Autodesk Inventor part; units mm, degrees
ref_plane "YZ Plane" through (0, 0, 0) normal (1, 0, 0) x (0, 1, 0)
ref_plane "XZ Plane" through (0, 0, 0) normal (0, 1, 0) x (-1, 0, 0)
ref_plane "XY Plane" through (0, 0, 0) normal (0, 0, 1) x (1, 0, 0)
sketch "Sketch1" plane through (0, 0, 0) normal (0, 1, 0) x (-1, 0, 0)
  line L0 (0, 0) -> (52.3748, 0) construction
  arc A0 (52.2043, -29.1712) -> (0.1705, -29.1712) centre (26.1874, -26.1874) ccw construction
  line L1 (0, 0) -> (-6.35, 0) construction
  line L2 (52.3748, 0) -> (58.7248, 0) construction
  line L3 (0, 0) -> (0, -26.1874) construction
  line L4 (52.3748, 0) -> (52.3748, -26.1874) construction
  line L5 (-3.175, 0) -> (0.1705, -29.1712)
  line L6 (55.5498, 0) -> (52.2043, -29.1712)
  arc A1 (0.1705, -29.1712) -> (52.2043, -29.1712) centre (26.1874, -26.1874) ccw
  line L7 (-0.0207, 3.5368) -> (52.3955, 3.5368)
  arc A2 (-0.0207, 3.5368) -> (-3.175, 0) centre (-0.0207, 0.3618) ccw
  arc A3 (55.5498, 0) -> (52.3955, 3.5368) centre (52.3955, 0.3618) ccw
  arc A4 (56.8115, -0.1447) -> (52.3955, 4.8068) centre (52.3955, 0.3618) ccw
  line L8 (52.3955, 4.8068) -> (-0.0207, 4.8068)
  arc A5 (-0.0207, 4.8068) -> (-4.4367, -0.1447) centre (-0.0207, 0.3618) ccw
  line L9 (-4.4367, -0.1447) -> (-1.0912, -29.3159)
  arc A6 (-1.0912, -29.3159) -> (53.466, -29.3159) centre (26.1874, -26.1874) ccw
  line L10 (56.8115, -0.1447) -> (53.466, -29.3159)
  dimension "d0" = 52.3748
  dimension "d1" = 52.3748
  dimension "d2" = 6.35
  dimension "d3" = 6.35
  dimension "d4" = 3.175
  dimension "d5" = 1.27
  dimension "d6" = 1.27
  dimension "d7" = 1.27
  dimension "d8" = 1.27
extrude "Extrusion1" add sketch "Sketch1" along normal blind 5.08
properties part number "Clippard Zip Tie 2" material "ABS Plastic"
Model file for the job. Use its own axes, mm. A direction names the side the tool comes from. Round coordinates to 2 decimals unless told otherwise and drop trailing zeros. Loops run counter-clockwise (first coordinate to the right, second up) from the corner with the lowest first, then second, coordinate; pieces in that order, holes last.
1. Band-saw the part on C-C, the plane z = -3.5. List the corners of the cut face in (x, y).
Check values:
outline: (-56.43, 0) - (-55.15, 0) - (-55.15, 5.08) - (-56.43, 5.08) - close; (2.77, 0) - (4.05, 0) - (4.05, 5.08) - (2.77, 5.08) - close
2. Wall check: probe 1 along X at (y, z) = (2.25, -38.5); probe 2 along X at (y, z) = (3.9, -13); probe 3 along Z at (x, y) = (-39, 0.25). Give the ranges that are in metal, low to high.
Check values:
probe 1: x = -50.73 to -49.3, -3.08 to -1.65
probe 2: x = -55.34 to -54.06, 1.68 to 2.96
probe 3: z = -50.47 to -49.03, 3.54 to 4.81
3. Mould opens along Z. For faces 1 (the flat face through (-26, 0, 4)), 2 (the cylindrical face through (-26.75, 2.5, -53.64)), 3 (the cylindrical face through (-26.72, 2.5, -52.37)) say: +Z half, -Z half, draft (parallel to the pull), parting line (faces both ways), or undercut.
Check values:
face 1: draft
face 2: -Z half
face 3: undercut
4. Band-saw the part on B-B, the plane y = 1.7. List the corners of the cut face in (x, z) (1 decimal).
Check values:
outline: (-56.8, -0.1) - (-53.5, -29.3) arc R27.5 ccw to (1.1, -29.3) - (4.4, -0.1) arc R4.4 ccw to (0, 4.8) - (-52.4, 4.8) arc R4.4 ccw to start; hole (-55.5, 0) - (-52.2, -29.2) arc R26.2 ccw to (-0.2, -29.2) - (3.2, 0) arc R3.2 ccw to (0, 3.5) - (-52.4, 3.5) arc R3.2 ccw to start
5. Band-saw the part on A-A, the plane x = -31.5. List the corners of the cut face in (y, z), and give its area (3 significant figures).
Check values:
outline: (0, -53.13) - (5.08, -53.13) - (5.08, -51.83) - (0, -51.83) - close; (0, 3.54) - (5.08, 3.54) - (5.08, 4.81) - (0, 4.81) - close
area: 13.0 mm2
6. Drop a flat-ended pin along its axis: P1, Ø2.5, axis at x = -16.5, y = 2.5, coming from the -Z side. Give the stop position or say it passes through.
Check values:
P1: stops at z = -52.32
7. Tool access for faces 4 (the cylindrical face through (2.41, 2.5, 2.45)), 5 (the flat face through (-55.16, 2.5, -14.53)): list every direction of +Z, -Z, +X, -X, +Y, -Y with a clear straight run to the whole face (end or side of a thin tool).
Check values:
face 4: +Y, -Y
face 5: -Z, -X, +Y, -Y
